Can you work these out from the drawing? Everything is in mm from the part's minimum corner. Give positions to 0.01 mm unless a question says otherwise; leave off trailing zeros. Order: outer loops, then holes, each group sorted by start corner. A loop starts at its lowest first (then second) coordinate and runs counter-clockwise, first axis right, second up. Notation, with made-up numbers: (51.5, 0.5) -> (79.5, 0.5) arc R26 ccw to (79.5, 37.5) -> close; hole circle Ø2 at (71.5, 88.25). An arc over 180 degrees is marked (long way). One line per item, written item: value.
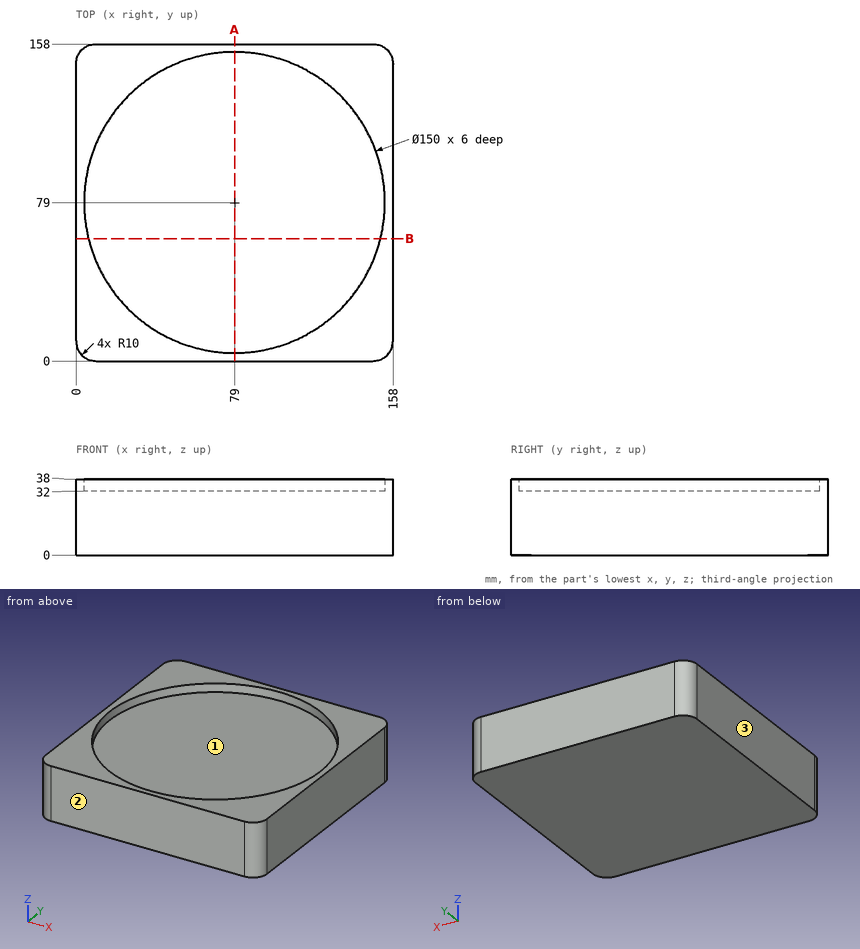
1) If I drill on line 1 along Y through (x, z) = (79, 34.5); line 2 along Z through (x, y) = (132, 52), over which ranges is the centre line in solid material (lowest first)?
Answer below:
line 1: y = 0 to 4, 154 to 158
line 2: z = 0 to 32
2) For P1, Ø1.5, axis at x = 141.5, y = 60, coming from the +Z side; P2, Ø1, axis at x = 21.5, z = 15, coming from the -Y side, each with a flat end and sliding along its axis, tell me the tip position at first contact or that it passes through.
Answer below:
P1: stops at z = 32
P2: stops at y = 0
3) Suppose I cut it at A-A, the plane x = 79. Write out the boundary of the cut face in (y, z).
Answer below:
outline: (0, 0) -> (158, 0) -> (158, 38) -> (154, 38) -> (154, 32) -> (4, 32) -> (4, 38) -> (0, 38) -> close
4) Suppose I cut it at B-B, the plane y = 61. Write out the boundary of the cut face in (x, z).
Answer below:
outline: (0, 0) -> (158, 0) -> (158, 38) -> (151.81, 38) -> (151.81, 32) -> (6.19, 32) -> (6.19, 38) -> (0, 38) -> close
5) We'd pull the mould along Y, two halves only. Please class the marked faces 1, 2 and 3: +Y half, -Y half, draft (parallel to the pull), parting line (faces both ways), or undercut.
Answer below:
face 1: undercut
face 2: -Y half
face 3: draft
